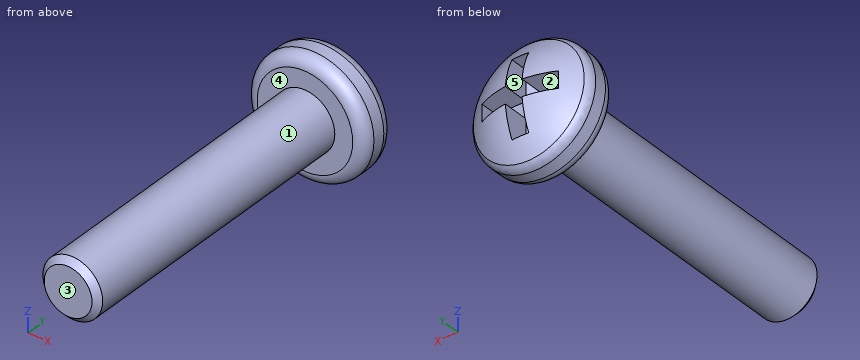
Autodesk Inventor part; units mm, degrees
ref_plane "Work Plane1" through (0, 29.9, 0) normal (0, -1, 0) x (1, 0, 0)
ref_plane "YZ Plane" through (0, 0, 0) normal (1, 0, 0) x (0, 1, 0)
ref_plane "XZ Plane" through (0, 0, 0) normal (0, 1, 0) x (-1, 0, 0)
sketch "Sketch1" plane through (0, 0, 0) normal (0, 0, 1) x (1, 0, 0)
  line L0 (0, 0) -> (0, 25.4)
  line L1 (2.5, 25.4) -> (2.5, 0)
  line L2 (2.5, 0) -> (0, 0)
  line L3 (0, 25.4) -> (0, 29.9)
  arc A0 (5, 27.9) -> (0, 29.9) centre (0, 22.65) ccw
  line L4 (2.5, 25.4) -> (5, 25.4)
  line L5 (-9.3694, 47.064) -> (8.7897, 47.064) construction
  line L6 (8.7897, 47.064) -> (8.7897, -18.3846) construction
  line L7 (8.7897, -18.3846) -> (-9.3694, -18.3846) construction
  line L8 (-9.3694, -18.3846) -> (-9.3694, 47.064) construction
  line L9 (5, 25.4) -> (5, 27.9)
  dimension "d0" = 25.4
  dimension "d1" = 2.5
  dimension "d2" = 4.5
  dimension "d4" = 2.5
  dimension "d31" = 2.5
  dimension "d33" = 2.5
revolve "Revolution1" add sketch "Sketch1" angle 360 about axis through (0, 0, 0) along (0, 1, 0)
chamfer "Chamfer1" distance 0.5 angle 45 1 edges at (-2.5, 0, 0)
fillet "Fillet1" radius 1 2 edges at (-5, 25.4, 0) (-5, 27.9, 0)
ref_plane "Work Plane1" through (0, 29.9, 0) normal (0, -1, 0) x (1, 0, 0)
sketch "Sketch4" plane through (0, 29.9, 0) normal (0, -1, 0) x (1, 0, 0)
  line L0 (0.7, 0.7) -> (0.7, 3.2)
  line L1 (0.7, 3.2) -> (-0.7, 3.2)
  line L2 (-0.7, 3.2) -> (-0.7, 0.7)
  line L3 (0.7, 0.7) -> (3.2, 0.7)
  line L4 (3.2, 0.7) -> (3.2, -0.7)
  line L5 (3.2, -0.7) -> (0.7, -0.7)
  line L6 (0.7, -0.7) -> (0.7, -3.2)
  line L7 (0.7, -3.2) -> (-0.7, -3.2)
  line L8 (-0.7, -3.2) -> (-0.7, -0.7)
  line L9 (-0.7, -0.7) -> (-3.2, -0.7)
  line L10 (-3.2, -0.7) -> (-3.2, 0.7)
  line L11 (-3.2, 0.7) -> (-0.7, 0.7)
  point P0 (0, 0)
  dimension "d57" = 2.5
  dimension "d58" = 1.4
  dimension "d59" = 2.5
  dimension "d60" = 1.4
  dimension "d61" = 2.5
  dimension "d62" = 2.5
  dimension "d63" = 1.4
  dimension "d64" = 90
  dimension "d65" = 2.5
  dimension "d66" = 1.4
  dimension "d67" = 90
extrude "Extrusion1" cut sketch "Sketch4" along normal blind 3
chamfer "Chamfer2" distance 0.7 angle 45 12 edges at (0.7, 26.9, -1.95) (0, 26.9, -3.2) (-0.7, 26.9, -1.95) (-1.95, 26.9, -0.7) (-3.2, 26.9, 0) (-1.95, 26.9, 0.7) (-0.7, 26.9, 1.95) (1.95, 26.9, -0.7) (3.2, 26.9, 0) (1.95, 26.9, 0.7) (0.7, 26.9, 1.95) (0, 26.9, 3.2)
properties part number "pan_head_screw" material "Stainless Steel, Polished"
Check sheet for the modelled part. Datum: model origin and axes. Units: mm. Face numbers are marked on the shaded views. A direction names the side the tool comes from. Round coordinates to 2 decimals unless told otherwise and drop trailing zeros. Loops run counter-clockwise (first coordinate to the right, second up) from the corner with the lowest first, then second, coordinate; pieces in that order, holes last. Notation, with made-up numbers: (36, -5) - (62, -5) arc R4 cw to (62, 2) - close; hole circle Ø2 at (77, 36.5). An arc over 180 degrees is marked (long way). Answer as a JSON object with one key per item and string values. Group by question number.
Q1. Gauge pin test, flat ends, axial feed: P1, Ø0.7, axis at x = -1.5, y = 28.5, coming from the +Z side; P2, Ø1.5, axis at y = 28.5, z = 0, coming from the -X side; P3, Ø0.7, axis at x = 2, y = 29, coming from the -Z side. Record the tip position at first contact, or that the pin passes through.
Q2. Scan lines: line 1 along Z through (x, y) = (0.25, 27.75); line 2 along Z through (x, y) = (-1.5, 22); line 3 along Z through (x, y) = (-2.5, 27.5). Record each from-to range of solid material in increasing order. Write a range as [from, to].
Q3. Mould release check, pull along X, two halves, no side actions. Record for the marked faces 1, 2 and 3: released by +X, released by -X, zero draft, split by the parting line, or undercut.
Q4. Sectioned sample at A-A, the plane y = 2.5. Enter the section's corners in (x, z).
Q5. Set-up check for the marked faces 4 and 5: record each of +Z, -Z, +X, -X, +Y, -Y from which the full face is reachable in a straight line by a thin tool's end or side.
Solution:
{
 "1": {"P1": "stops at z = 4.49", "P2": "stops at x = -4.95", "P3": "stops at z = -3.57"},
 "2": {"line 1": "z = [-4.95, -3.2], [3.2, 4.95]", "line 2": "z = [-2, 2]", "line 3": "z = [-4.33, -0.6], [0.6, 4.33]"},
 "3": {"face 1": "split by the parting line", "face 2": "undercut", "face 3": "zero draft"},
 "4": {"outline": "circle Ø5 at (0, 0)"},
 "5": {"face 4": "-Y", "face 5": "+Y"}
}
